Design review of the part built by this model. Coordinates are the model's own, in mm. A direction names the side the tool comes from. Round coordinates to 2 decimals unless told otherwise and drop trailing zeros. Loops run counter-clockwise (first coordinate to the right, second up) from the corner with the lowest first, then second, coordinate; pieces in that order, holes last. Notation, with made-up numbers: (48.5, -23.75) - (71.5, -23.75) arc R30 ccw to (71.5, 15.25) - close; hole circle Ø11 at (36, -9). An arc over 180 degrees is marked (long way). Use one line per item in the form item = value. Start each with the question number.
(1) The part is to be moulded in two halves that separate along X. For faces 3 (the flat face through (0, 12.7, 0)), 4 (the flat face through (-6.142, 0, 0)), 5 (the flat face through (0, 0, 1.008)), 6 (the flat face through (6.142, 0, 0)), say which applies: released by +X, released by -X, zero draft, split by the parting line, or undercut.
(2) Wall thickness on probe 1 along Z at (x, y) = (-1.25, -3.5): over which ranges is the line inside the solid? List them lowest first. Write a range as [from, to].
(3) For pin 1 (5 mm diameter, centred on x = 0.5, y = 7.5, fed in from +Z), flat-tipped, find the tip position at first contact; note if it passes through.
(4) Machinability: for faces 1 (the flat face through (0, -12.7, 0)), 2 (the flat face through (0, 0, -1.008)), which of the approach directions +Z, -Z, +X, -X, +Y, -Y give a long, thin tool a straight path to every point of the face, cutting with its end or side? Answer none if there is none.
(5) We need section B-B, the plane x = -5.5. Write out the cut boundary in (y, z).
from build123d import *

# Parameters (mm, degrees)
F1_DEPTH = 12.7


with BuildPart() as f1:
    # F0 (on Front) → F1 (new body, symmetric)
    with BuildSketch(Plane.XZ):
        with BuildLine():
            Line((-5.73532, -1.00838), (5.73532, -1.00838))
            ThreePointArc((5.73532, -1.00838), (5.749638, -1.00919), (5.763773, -1.011608))
            Line((5.763773, -1.011608), (5.892995, -1.041315))
            ThreePointArc((5.892995, -1.041315), (6.065089, -1.002247), (6.14172, -0.84328))
            Line((6.14172, -0.84328), (6.14172, 0.84328))
            ThreePointArc((6.14172, 0.84328), (6.065089, 1.002247), (5.892995, 1.041315))
            Line((5.892995, 1.041315), (5.763773, 1.011608))
            ThreePointArc((5.763773, 1.011608), (5.749638, 1.00919), (5.73532, 1.00838))
            Line((5.73532, 1.00838), (-5.73532, 1.00838))
            ThreePointArc((-5.73532, 1.00838), (-5.749638, 1.00919), (-5.763773, 1.011608))
            Line((-5.763773, 1.011608), (-5.892995, 1.041315))
            ThreePointArc((-5.892995, 1.041315), (-6.065089, 1.002247), (-6.14172, 0.84328))
            Line((-6.14172, 0.84328), (-6.14172, -0.84328))
            ThreePointArc((-6.14172, -0.84328), (-6.065089, -1.002247), (-5.892995, -1.041315))
            Line((-5.892995, -1.041315), (-5.763773, -1.011608))
            ThreePointArc((-5.763773, -1.011608), (-5.749638, -1.00919), (-5.73532, -1.00838))
        make_face()
    extrude(amount=F1_DEPTH, both=True)


solid = f1.part
Data:
q1.face_3 = zero draft
q1.face_4 = released by -X
q1.face_5 = undercut
q1.face_6 = released by +X
q2.probe_1 = [-1.01, 1.01]
q3.pin_1 = 1.01
q4.face_1 = +Z, -Z, +X, -X, -Y
q4.face_2 = -Z, +Y, -Y
q5.outline = (-12.7, -1.01) - (12.7, -1.01) - (12.7, 1.01) - (-12.7, 1.01) - close
